Check sheet for the modelled part. Datum: model origin and axes. Units: mm. Give positions to 0.01 mm unless a question says otherwise; leave off trailing zeros. Loops run counter-clockwise (first coordinate to the right, second up) from the corner with the lowest first, then second, coordinate; pieces in that order, holes last. Notation, with made-up numbers: (-17.5, 63) -> (20.5, 63) arc R21 cw to (20.5, 98) -> close; hole circle Ø8 at (-27, 80). An arc over 180 degrees is marked (long way). Write each question's results on one line, items separated by ' | '. Start each with the question number.
1. Cross-section at D-D on x = 0. Record the boundary of the cut face in (y, z).
2. Cross-section at C-C on z = 1.75. Count the separate pieces of the cut face and the enclosed holes in it, and give its area (3 significant figures).
3. Gauge pin test, flat end, axial feed: pin 1 Ø2 at (x, z) = (-2.5, 1.5) entering from -Y. Record the tip position at first contact, or that the pin passes through.
4. Cross-section at A-A on x = -60. Record the boundary of the cut face in (y, z), and give its area (3 significant figures).
5. Cross-section at B-B on y = 69. Record the boundary of the cut face in (x, z).
6. Material ranges on L1, parallel to X at y = 81, z = 3.25; L2, parallel to X at y = 79, z = 3.75; L3, parallel to Y at x = -62, z = 2, recorded low to high. Write a range as from..to.
from build123d import *

# Parameters (mm, degrees)
EXTRUSION1_DEPTH = 6.35
HOLE1_D          = 6.35


with BuildPart() as part:
    # Sketch1 → Extrusion1 (new body)
    with BuildSketch(Plane.XY):
        Polygon((-72.704579377, 193.412844037), (-72.704579377, 91.812844037), (28.895420623, -9.787155963), (130.495420623, -9.787155963), (130.495420623, 193.412844037), align=None)
    extrude(amount=EXTRUSION1_DEPTH)

    # Hole1 (through all)
    with Locations(Plane.XY.offset(6.35)):
        with Locations((-60.004579377, 180.712844037), (-34.604579377, 180.712844037), (-60.004579377, 155.312844037), (-34.604579377, 155.312844037), (-60.004579377, 129.912844037), (-34.604579377, 129.912844037), (-60.004579377, 104.512844037), (-34.604579377, 104.512844037), (117.795420623, 79.112844037), (117.795420623, 53.712844037), (92.395420623, 79.112844037), (92.395420623, 53.712844037), (-9.204579377, 180.712844037), (-9.204579377, 155.312844037), (-9.204579377, 129.912844037), (-9.204579377, 104.512844037), (16.195420623, 180.712844037), (16.195420623, 155.312844037), (16.195420623, 129.912844037), (16.195420623, 104.512844037), (41.595420623, 180.712844037), (41.595420623, 155.312844037), (41.595420623, 129.912844037), (41.595420623, 104.512844037), (66.995420623, 180.712844037), (66.995420623, 155.312844037), (66.995420623, 129.912844037), (66.995420623, 104.512844037), (92.395420623, 180.712844037), (92.395420623, 155.312844037), (92.395420623, 129.912844037), (92.395420623, 104.512844037), (117.795420623, 180.712844037), (117.795420623, 155.312844037), (117.795420623, 129.912844037), (117.795420623, 104.512844037), (117.795420623, 28.312844037), (92.395420623, 28.312844037), (117.795420623, 2.912844037), (92.395420623, 2.912844037), (66.995420623, 79.112844037), (66.995420623, 53.712844037), (66.995420623, 28.312844037), (66.995420623, 2.912844037), (41.595420623, 79.112844037), (41.595420623, 53.712844037), (41.595420623, 28.312844037), (41.595420623, 2.912844037)):
            Hole(HOLE1_D / 2)


solid = part.part
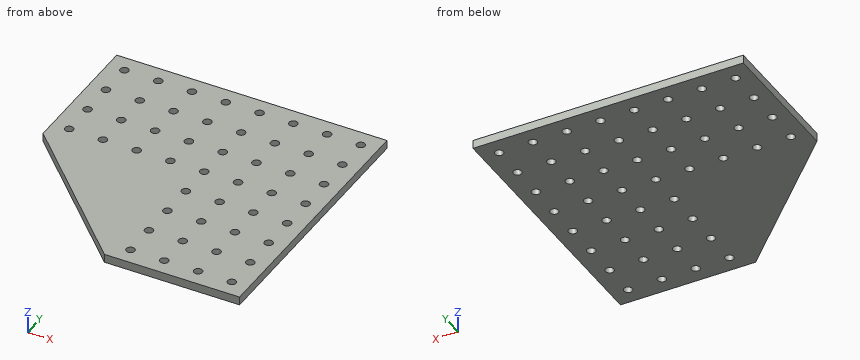
Geometry says:
1) outline: (19.11, 0) -> (193.41, 0) -> (193.41, 6.35) -> (19.11, 6.35) -> close
2) separate pieces: 1 | enclosed holes: 48 | area: 34,600 mm^2
3) pin 1: y = 20.61
4) outline: (79.11, 0) -> (101.34, 0) -> (101.34, 6.35) -> (79.11, 6.35) -> close; (107.69, 0) -> (126.74, 0) -> (126.74, 6.35) -> (107.69, 6.35) -> close; (133.09, 0) -> (152.14, 0) -> (152.14, 6.35) -> (133.09, 6.35) -> close; (158.49, 0) -> (177.54, 0) -> (177.54, 6.35) -> (158.49, 6.35) -> close; (183.89, 0) -> (193.41, 0) -> (193.41, 6.35) -> (183.89, 6.35) -> close | area: 565 mm^2
5) outline: (-49.89, 0) -> (130.5, 0) -> (130.5, 6.35) -> (-49.89, 6.35) -> close
6) L1: -61.89..39.04, 44.15..64.44, 69.55..89.84, 94.95..115.24, 120.35..130.5 | L2: -59.89..38.42, 44.77..63.82, 70.17..89.22, 95.57..114.62, 120.97..130.5 | L3: 81.11..102.04, 106.98..127.44, 132.38..152.84, 157.78..178.24, 183.18..193.41
